from build123d import *

# Parameters (mm, degrees)
SKETCH1_R               = 76.1365
BOSS_EXTRUDE1_DEPTH     = 203.2
CHAMFER1_SIZE           = 2.032
CUT_EXTRUDE2_DEPTH      = 230.964721782
CUT_EXTRUDE2_DEPTH_BACK = 230.964721782
F_1_4_CLEARANCE_HOLE1_D = 6.7564
SKETCH6_R               = 15.875
CUT_EXTRUDE3_DEPTH      = 15.875
CHAMFER2_SIZE           = 2.54


with BuildPart() as part:
    # Sketch1 → Boss-Extrude1 (new body)
    with BuildSketch(Plane(origin=(0, 0, 0), x_dir=(1, 0, 0), z_dir=(0, 1, 0))):
        with Locations(Location((0, 0, 0), (0, 0, 270))):
            Circle(SKETCH1_R)
    extrude(amount=BOSS_EXTRUDE1_DEPTH)

    # Chamfer1
    chamfer1_edges = [part.edges().sort_by_distance(p)[0] for p in [
        (0, 0, -76.1365),
        (0, 203.2, -76.1365),
    ]]
    chamfer(chamfer1_edges, length=CHAMFER1_SIZE)

    # Sketch3 → Cut-Extrude2 (cut, two sides: drawn at the far end of the back side and taken through both)
    with BuildSketch(Plane(origin=(0, 203.2, 0), x_dir=(1, 0, 0), z_dir=(0, 1, 0)).offset(-CUT_EXTRUDE2_DEPTH_BACK)):
        with BuildLine():
            Line((-7.6470512, 24.221531908), (-22.225, 59.415813613))
            ThreePointArc((-22.225, 59.415813613), (0, 63.4365), (22.225, 59.415813613))
            Line((22.225, 59.415813613), (7.6470512, 24.221531908))
            ThreePointArc((7.6470512, 24.221531908), (0, 25.4), (-7.6470512, 24.221531908))
        make_face()
        with BuildLine():
            Line((24.221531908, 7.6470512), (59.415813613, 22.225))
            ThreePointArc((59.415813613, 22.225), (63.4365, 0), (59.415813613, -22.225))
            Line((59.415813613, -22.225), (24.221531908, -7.6470512))
            ThreePointArc((24.221531908, -7.6470512), (25.4, 0), (24.221531908, 7.6470512))
        make_face()
        with BuildLine():
            Line((7.6470512, -24.221531908), (22.225, -59.415813613))
            ThreePointArc((22.225, -59.415813613), (0, -63.4365), (-22.225, -59.415813613))
            Line((-22.225, -59.415813613), (-7.6470512, -24.221531908))
            ThreePointArc((-7.6470512, -24.221531908), (0, -25.4), (7.6470512, -24.221531908))
        make_face()
        with BuildLine():
            Line((-24.221531908, -7.6470512), (-59.415813613, -22.225))
            ThreePointArc((-59.415813613, -22.225), (-63.4365, 0), (-59.415813613, 22.225))
            Line((-59.415813613, 22.225), (-24.221531908, 7.6470512))
            ThreePointArc((-24.221531908, 7.6470512), (-25.4, 0), (-24.221531908, -7.6470512))
        make_face()
    extrude(amount=CUT_EXTRUDE2_DEPTH + CUT_EXTRUDE2_DEPTH_BACK, mode=Mode.SUBTRACT)

    # 1/4 Clearance Hole1 (through all)
    with Locations(Plane(origin=(0, 203.2, 0), x_dir=(1, 0, 0), z_dir=(0, 1, 0))):
        with Locations((0, 0)):
            Hole(F_1_4_CLEARANCE_HOLE1_D / 2)

    # Sketch6 → Cut-Extrude3 (cut)
    with BuildSketch(Plane.XZ):
        with Locations(Location((0, 0, 0), (0, 0, 270))):
            Circle(SKETCH6_R)
    extrude(amount=-CUT_EXTRUDE3_DEPTH, mode=Mode.SUBTRACT)

    # Chamfer2
    chamfer2_edges = [part.edges().sort_by_distance(p)[0] for p in [
        (0, 0, 15.875),
    ]]
    chamfer(chamfer2_edges, length=CHAMFER2_SIZE)


solid = part.part
Work out the finished part from the listing and answer in its coordinate system (mm). A direction names the side the tool comes from. Coordinates: 2 decimals unless noted, no trailing zeros. Write each loop counter-clockwise with the first axis right and the second up, starting at its lowest first coordinate (ties: lowest second). Pieces come first, ordered by that corner, then holes. Notation, with made-up numbers: M 46.5,64 L 65.5,64 A15 cw 65.5,78 Z; hole C -36,65.5 d10. An arc over 180 degrees is marked long. Answer as CSV lines item,"result". Start each with the question number.
Item 1: Flat-ended cylindrical pins translate along their axes: P1, Ø8, axis at x = -12, y = 64, coming from the +Z side; P2, Ø11, axis at x = 0, z = 0, coming from the +Y side; P3, Ø10, axis at y = 136.5, z = 26, coming from the -X side; P4, Ø12, axis at x = 45, y = 143, coming from the -Z side. Find the tip coordinate at first contact, or state that the pin passes through.
Item 2: Section A-A on x = 0 is taken. Write down the section's boundary in (y, z) (1 decimal), and give its area (3 significant figures).
Item 3: Consider L1, parallel to Z at x = 15.5, y = 96; L2, parallel to X at y = 14, z = 4; L3, parallel to X at y = 176, z = -34.5. Determine where each line is inside the solid, lowest interval first.
Item 4: Section B-B on z = 0 is taken. Write down the section's boundary in (x, y) (1 decimal).
Item 5: A tool of negligible diameter and unlimited length cuts with its end or side. For faces 3 (the face through (4, 15.875, 0)), 4 (the face through (1, 203.2, 15)), 5 (the face through (-14.834, 100.178, -41.572)), from which of +Z, -Z, +X, -X, +Y, -Y can it reach the whole face along a straight path? Write none if from no direction.
Item 6: Determine the mould class of faces 1 (the face through (-15, 0, 15)), 2 (the face through (-41.572, 100.178, 14.834)) for opening direction X: released by +X, released by -X, zero draft, split by the parting line, or undercut.
Item 7: Section C-C on y = 138 is taken. Write down the section's boundary in (x, z) (1 decimal).
Checks:
1,P1,"stops at z = 75.72"
1,P2,"stops at y = 203.2"
1,P3,"stops at x = -73.18"
1,P4,"stops at z = -65.39"
2,outline,"M 0,-74.1 L 2,-76.1 L 201.2,-76.1 L 203.2,-74.1 L 203.2,-63.4 L 0,-63.4 Z; M 0,-25.4 L 203.2,-25.4 L 203.2,-3.4 L 15.9,-3.4 L 15.9,-15.9 L 2.5,-15.9 L 0,-18.4 Z; M 0,18.4 L 2.5,15.9 L 15.9,15.9 L 15.9,3.4 L 203.2,3.4 L 203.2,25.4 L 0,25.4 Z; M 0,63.4 L 203.2,63.4 L 203.2,74.1 L 201.2,76.1 L 2,76.1 L 0,74.1 Z"
2,area,"13,700 mm²"
3,L1,"z = -74.54 to -61.51, -43.18 to 43.18, 61.51 to 74.54"
3,L2,"x = -76.03 to -63.31, -25.08 to -15.36, 15.36 to 25.08, 63.31 to 76.03"
3,L3,"x = -67.87 to -11.9, 11.9 to 67.87"
4,outline,"M -76.1,2 L -74.1,0 L -63.4,0 L -63.4,203.2 L -74.1,203.2 L -76.1,201.2 Z; M -25.4,0 L -18.4,0 L -15.9,2.5 L -15.9,15.9 L -3.4,15.9 L -3.4,203.2 L -25.4,203.2 Z; M 3.4,15.9 L 15.9,15.9 L 15.9,2.5 L 18.4,0 L 25.4,0 L 25.4,203.2 L 3.4,203.2 Z; M 63.4,0 L 74.1,0 L 76.1,2 L 76.1,201.2 L 74.1,203.2 L 63.4,203.2 Z"
5,face 3,"-Y"
5,face 4,"+Z, -Z, +X, -X, +Y"
5,face 5,"+Y, -Y"
6,face 1,"zero draft"
6,face 2,"undercut"
7,outline,"C 0,0 d152.3; hole M -59.4,-22.2 L -24.2,-7.6 A25.4 cw -24.2,7.6 L -59.4,22.2 A63.4 ccw Z; hole M -22.2,-59.4 A63.4 ccw 22.2,-59.4 L 7.6,-24.2 A25.4 cw -7.6,-24.2 Z; hole M -22.2,59.4 L -7.6,24.2 A25.4 cw 7.6,24.2 L 22.2,59.4 A63.4 ccw Z; hole C 0,0 d6.8; hole M 24.2,-7.6 L 59.4,-22.2 A63.4 ccw 59.4,22.2 L 24.2,7.6 A25.4 cw Z"
